Source: CAD feature listing. Evaluate the final solid. Frame: model axes, mm. Face numbers are marked on the shaded views. A direction names the side the tool comes from. Give positions to 0.01 mm unless a question says otherwise; leave off trailing zeros. Loops run counter-clockwise (first coordinate to the right, second up) from the corner with the lowest first, then second, coordinate; pieces in that order, holes last. Notation, with made-up numbers: (-35, 40.25) -> (-24, 40.25) arc R26 cw to (-24, 66.25) -> close; hole circle Ø7 at (-31, 51.5). An arc over 180 degrees is marked (long way). Return JSON: item names as keys, results as strings. Group by question number.
(1) Ray query, line 1 (X direction, y = 13.5, z = -15); line 2 (Y direction, x = 51, z = -2.75); line 3 (Z direction, x = 56.5, y = 4). Return the intervals inside material, ascending. Write a range as from..to.
(2) Access query for the marked faces 5 and 6. Directions: +Z, -Z, +X, -X, +Y, -Y. A direction counts if a zero-diameter tool reaches every point of the face in a straight line with its end or side. Return the directions, or none.
(3) Cut plane C-C on z = -10.75. Return loops of the section in (x, y).
(4) Pin query (flat end, axial travel): pin 1 (3.5 mm diameter, centred on x = 64.5, y = 14, fed in from -Z); pin 2 (5 mm diameter, centred on y = 9, z = -7.5, fed in from +X); pin 3 (2 mm diameter, centred on x = 50, y = 10, fed in from -Z); pin 4 (10 mm diameter, centred on x = 43.5, y = 18.5, fed in from +Z). Return the tip coordinate at first contact, or that it passes through.
(5) Cut plane B-B on x = 42. Return loops of the section in (y, z), then the cut area to 3 significant figures.
(6) Cut plane A-A on y = 12. Return loops of the section in (x, z), then the cut area to 3 significant figures.
(7) Cut plane D-D on y = 16. Return loops of the section in (x, z), then the cut area to 3 significant figures.
(8) Draft query along X for the marked faces 1, 2, 3 and 4. Return one class per face: released by +X, released by -X, zero draft, split by the parting line, or undercut.
```python
from build123d import *

# Parameters (mm, degrees)
SKETCH_219_W                = 70
SKETCH_219_H                = 20
EXTRUDE_370_DEPTH           = 3
SKETCH_424_W                = 3
SKETCH_424_H                = 16
EXTRUDE_647_DEPTH           = 20
CUT_EXTRUDE_897_DEPTH       = 5
CUT_EXTRUDE_897_DEPTH_BACK  = 3
SKETCH_8_W                  = 3
SKETCH_8_H                  = 16
EXTRUDE_1252_DEPTH          = 20
CUT_EXTRUDE_1518_DEPTH      = 64
CUT_EXTRUDE_1518_DEPTH_BACK = 3
SKETCH_11_W                 = 56
SKETCH_11_H                 = 2.665153407
EXTRUDE_1792_DEPTH          = 7


with BuildPart() as part:
    # Sketch 219 → Extrude 370 (new body)
    with BuildSketch(Plane(origin=(0, 0, 0), x_dir=(1, 0, 0), z_dir=(0, 1, 0))):
        with Locations((35, 10)):
            Rectangle(SKETCH_219_W, SKETCH_219_H)
    extrude(amount=EXTRUDE_370_DEPTH)

    # Sketch 424 → Extrude 647 (add)
    with BuildSketch(Plane(origin=(0, 3, 0), x_dir=(1, 0, 0), z_dir=(0, 1, 0))):
        with Locations((5.5, 10)):
            Rectangle(SKETCH_424_W, SKETCH_424_H)
    extrude(amount=EXTRUDE_647_DEPTH)

    # Sketch 702 → Cut-Extrude 897 (cut, two sides)
    with BuildSketch(Plane.ZY.offset(-4)) as cut_extrude_897_sk:
        Polygon((-45.532064127, 82.064128255), (-16, 23), (-10, 11), (-4, 23), (25.532064127, 82.064128255), (25.532064127, 214.135534064), (-45.532064127, 214.135534064), align=None)
    extrude(amount=CUT_EXTRUDE_897_DEPTH, mode=Mode.SUBTRACT)
    extrude(cut_extrude_897_sk.sketch, amount=-CUT_EXTRUDE_897_DEPTH_BACK, mode=Mode.SUBTRACT)

    # Эскиз8 → Extrude 1252 (add)
    with BuildSketch(Plane(origin=(31.408501121, 3, 2.625790974), x_dir=(1, 0, 0), z_dir=(0, 1, 0))):
        with Locations((33.091498879, 12.625790974)):
            Rectangle(SKETCH_8_W, SKETCH_8_H)
    extrude(amount=EXTRUDE_1252_DEPTH)

    # Эскиз10 → Cut-Extrude 1518 (cut, two sides)
    with BuildSketch(Plane(origin=(63, 0, 2.625790974), x_dir=(0, 0, 1), z_dir=(-1, 0, 0))) as cut_extrude_1518_sk:
        Polygon((-48.157855101, 82.064128255), (-18.625790974, 23), (-12.625790974, 11), (-6.625790974, 23), (22.906273154, 82.064128255), (22.906273154, 214.135534064), (-48.157855101, 214.135534064), align=None)
    extrude(amount=CUT_EXTRUDE_1518_DEPTH, mode=Mode.SUBTRACT)
    extrude(cut_extrude_1518_sk.sketch, amount=-CUT_EXTRUDE_1518_DEPTH_BACK, mode=Mode.SUBTRACT)

    # Эскиз11 → Extrude 1792 (add)
    with BuildSketch(Plane(origin=(0, 3, 0), x_dir=(1, 0, 0), z_dir=(0, 1, 0))):
        with Locations((35, 10.036015586)):
            Rectangle(SKETCH_11_W, SKETCH_11_H)
    extrude(amount=EXTRUDE_1792_DEPTH)


solid = part.part
```
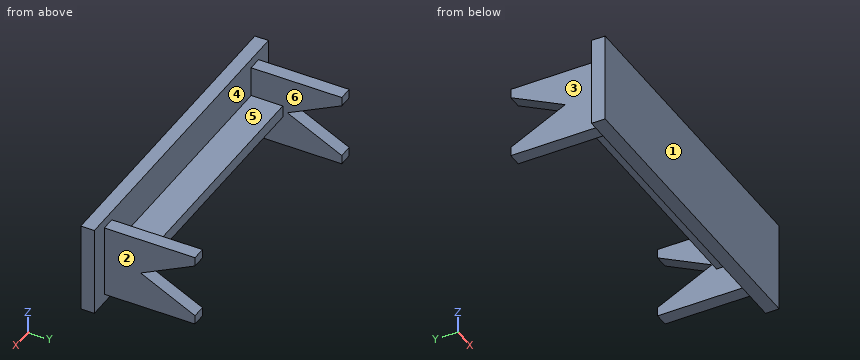
Answers:
{
 "1": {"line 1": "4..7, 63..66", "line 2": "0..3", "line 3": "-11.37..-8.7"},
 "2": {"face 5": "+Z, +Y", "face 6": "+Y"},
 "3": {"outline": "(0, 0) -> (70, 0) -> (70, 3) -> (66, 3) -> (66, 12.5) -> (63, 12.5) -> (63, 10) -> (7, 10) -> (7, 12.5) -> (4, 12.5) -> (4, 3) -> (0, 3) -> close"},
 "4": {"pin 1": "z = -18", "pin 2": "x = 66", "pin 3": "z = -11.37", "pin 4": "through"},
 "5": {"outline": "(0, -20) -> (3, -20) -> (3, -11.37) -> (10, -11.37) -> (10, -8.7) -> (3, -8.7) -> (3, 0) -> (0, 0) -> close", "area": "78.7 mm²"},
 "6": {"outline": "(4, -18) -> (7, -18) -> (7, -10.5) -> (4, -10.5) -> close; (4, -9.5) -> (7, -9.5) -> (7, -2) -> (4, -2) -> close; (63, -18) -> (66, -18) -> (66, -10.5) -> (63, -10.5) -> close; (63, -9.5) -> (66, -9.5) -> (66, -2) -> (63, -2) -> close", "area": "90.0 mm²"},
 "7": {"outline": "(4, -18) -> (7, -18) -> (7, -12.5) -> (4, -12.5) -> close; (4, -7.5) -> (7, -7.5) -> (7, -2) -> (4, -2) -> close; (63, -18) -> (66, -18) -> (66, -12.5) -> (63, -12.5) -> close; (63, -7.5) -> (66, -7.5) -> (66, -2) -> (63, -2) -> close", "area": "66.0 mm²"},
 "8": {"face 1": "zero draft", "face 2": "released by +X", "face 3": "released by -X", "face 4": "undercut"}
}
